```python
from build123d import *

# Parameters (mm, degrees)
SKETCH1_W           = 69.85
SKETCH1_H           = 25.4
SKETCH1_R           = 5.3975
BOSS_EXTRUDE1_DEPTH = 31.75
SKETCH2_W           = 71.374
SKETCH2_H           = 20.955
CUT_EXTRUDE1_DEPTH  = 22.86
SKETCH2_3_W         = 5.08
SKETCH2_3_H         = 5.588
CUT_EXTRUDE2_DEPTH  = 13.462
SKETCH3_R           = 1.5875
CUT_EXTRUDE3_DEPTH  = 9.89
SKETCH8_R           = 1.5875
BOSS_EXTRUDE2_DEPTH = 2.54


with BuildPart() as part:
    # Sketch1 → Boss-Extrude1 (new body)
    with BuildSketch(Plane(origin=(0, 0, 0), x_dir=(0, 0, -1), z_dir=(1, 0, 0))):
        with Locations((22.225, 0)):
            Rectangle(SKETCH1_W, SKETCH1_H)
        Circle(SKETCH1_R, mode=Mode.SUBTRACT)
    extrude(amount=BOSS_EXTRUDE1_DEPTH)

    # Sketch2 → Cut-Extrude1 (cut)
    with BuildSketch(Plane.ZY):
        with Locations((-24.003, 0)):
            Rectangle(SKETCH2_W, SKETCH2_H)
    extrude(amount=-CUT_EXTRUDE1_DEPTH, mode=Mode.SUBTRACT)

    # Sketch2_3 → Cut-Extrude2 (cut)
    with BuildSketch(Plane.ZY):
        with Locations((14.224, 0)):
            Rectangle(SKETCH2_3_W, SKETCH2_3_H)
    extrude(amount=-CUT_EXTRUDE2_DEPTH, mode=Mode.SUBTRACT)

    # Sketch3 → Cut-Extrude3 (cut, through all)
    with BuildSketch(Plane.ZY.offset(-22.86)):
        with Locations((-53.975, 6.35)):
            Circle(SKETCH3_R)
        with Locations((-53.975, -6.35)):
            Circle(SKETCH3_R)
    extrude(amount=-CUT_EXTRUDE3_DEPTH, mode=Mode.SUBTRACT)

    # Sketch8 → Boss-Extrude2 (add)
    with BuildSketch(Plane(origin=(31.75, 0, 0), x_dir=(0, 0, -1), z_dir=(1, 0, 0))):
        with Locations((53.975, -6.35)):
            Circle(SKETCH8_R)
        with Locations((53.975, 6.35)):
            Circle(SKETCH8_R)
    extrude(amount=-BOSS_EXTRUDE2_DEPTH)


solid = part.part
```
Build history of the part. All positions in model axes, mm. A direction names the side the tool comes from. Give positions to 0.01 mm unless a question says otherwise; leave off trailing zeros. Loops run counter-clockwise (first coordinate to the right, second up) from the corner with the lowest first, then second, coordinate; pieces in that order, holes last.
1) Band-saw the part on C-C on z = 0. List the corners of the cut face in (x, y), then the cut area to 3 significant figures.
Values follow:
outline: (0, -12.7) - (31.75, -12.7) - (31.75, -5.4) - (22.86, -5.4) - (22.86, -10.48) - (0, -10.48) - close; (0, 10.48) - (22.86, 10.48) - (22.86, 5.4) - (31.75, 5.4) - (31.75, 12.7) - (0, 12.7) - close
area: 231 mm2
2) Probe line 1 along Y through (x, z) = (4, -42); line 2 along Z through (x, y) = (26.5, -6.35); line 3 along X through (y, z) = (7, -14). List the from-to ranges inside material, lowest first.
Values follow:
line 1: y = -12.7 to -10.48, 10.48 to 12.7
line 2: z = -57.15 to -55.56, -52.39 to 12.7
line 3: x = 22.86 to 31.75
3) Two-plate mould, pull along Y, no slides. Class faces 1 (the face through (14, 0, 11.684)), 2 (the face through (0, 12, -22)), 3 (the face through (16, 12.7, -22)), 4 (the face through (29.21, 6, -54)): released by +Y, released by -Y, zero draft, split by the parting line, or undercut.
Values follow:
face 1: undercut
face 2: zero draft
face 3: released by +Y
face 4: undercut
4) Band-saw the part on A-A on y = 0. List the corners of the cut face in (x, z), then the cut area to 3 significant figures.
Values follow:
outline: (13.46, 11.68) - (22.86, 11.68) - (22.86, 5.4) - (31.75, 5.4) - (31.75, 12.7) - (13.46, 12.7) - close; (22.86, -57.15) - (31.75, -57.15) - (31.75, -5.4) - (22.86, -5.4) - close
area: 535 mm2
5) 3-axis set-ups, long thin cutter, end or side, ignore diameter. For faces 5 (the face through (16, 0, 12.7)), 6 (the face through (25.99, 5.38, -55.23)), 7 (the face through (11, -10.478, -23)): which of +Z, -Z, +X, -X, +Y, -Y reach the whole face in a straight line?
Values follow:
face 5: +Z, +X, -X, +Y, -Y
face 6: -X
face 7: -Z, -X
6) Drop flat-ended pins along their axis: P1, Ø10.5, axis at y = 1.5, z = -26.5, coming from the -X side; P2, Ø1.1, axis at y = 1, z = 12, coming from the -X side; P3, Ø12, axis at x = 3.5, y = -5.5, coming from the -Z side. Give the stop position or say it passes through.
Values follow:
P1: stops at x = 22.86
P2: stops at x = 13.46
P3: stops at z = -57.15
7) Band-saw the part on B-B on x = 8. List the corners of the cut face in (y, z).
Values follow:
outline: (-12.7, -57.15) - (-10.48, -57.15) - (-10.48, 11.68) - (-2.79, 11.68) - (-2.79, 12.7) - (-12.7, 12.7) - close; (2.79, 11.68) - (10.48, 11.68) - (10.48, -57.15) - (12.7, -57.15) - (12.7, 12.7) - (2.79, 12.7) - close
8) Band-saw the part on D-D on x = 25. State how many separate pieces and enclosed holes the cut face has, then the cut area to 3 significant figures.
Values follow:
separate pieces: 1
enclosed holes: 3
area: 1,670 mm2
